Autodesk Inventor part; units mm, degrees
ref_plane "YZ Plane" through (0, 0, 0) normal (1, 0, 0) x (0, 1, 0)
ref_plane "XZ Plane" through (0, 0, 0) normal (0, 1, 0) x (-1, 0, 0)
ref_plane "XY Plane" through (0, 0, 0) normal (0, 0, 1) x (1, 0, 0)
sketch "Sketch1" plane through (0, 0, 0) normal (0, 1, 0) x (-1, 0, 0)
  line L0 (50, -20) -> (-50, -20)
  line L1 (-50, -20) -> (-50, 60)
  line L2 (-50, 60) -> (50, 60)
  line L3 (50, 60) -> (50, -20)
  point P0 (0, 0)
  dimension "d0" = 100
  dimension "d1" = 80
  dimension "d2" = 20
  dimension "d3" = 50
extrude "Plate1" add sketch "Sketch1" along normal blind 3
sketch "Sketch3" plane through (0, 3, 0) normal (0, 1, 0) x (1, 0, 0)
  circle A0 centre (9.405, -34) radius 1.05
  circle A1 centre (9.405, -6) radius 1.05
  circle A2 centre (0, -34) radius 1.05
  circle A3 centre (0, -6) radius 1.05
  circle A4 centre (-9.405, -34) radius 1.05
  circle A5 centre (-9.405, -6) radius 1.05
  line L0 (15.405, 0) -> (15.405, -40)
  line L1 (-15.405, -40) -> (15.405, -40)
  line L2 (-15.405, -40) -> (-15.405, 0)
  line L3 (15.405, 0) -> (-15.405, 0)
  point P0 (0, 0)
hole "Hole1" at (-9.405, 3, 6) at (0, 3, 6) at (9.405, 3, 6) at (9.405, 3, 34) at (0, 3, 34) at (-9.405, 3, 34) direction (0, -1, 0) diameter 2.1 depth 3 countersink diameter 4 countersink angle 90
equation "\"d20\" = Thickness"
equation "\"d4\" = Thickness"
equation "\"BendReliefWidth\" = Thickness"
equation "\"BendReliefDepth\" = 0.5 * Thickness"
equation "\"CornerReliefSize\" = 4 * Thickness"
equation "\"MinimumRemnant\" = 2 * Thickness"
equation "\"TransitionRadius\" = BendRadius"
equation "\"JacobiRadiusSize\" = BendRadius"
equation "\"GapSize\" = Thickness"
properties part number "axis_12_bottom_frame(bottom)" material "Aluminum 6061-AHC"
Input: part model. Units: mm. Frame: model coordinates. Coordinates: 2 decimals unless noted, no trailing zeros. Write each loop counter-clockwise with the first axis right and the second up, starting at its lowest first coordinate (ties: lowest second). Pieces come first, ordered by that corner, then holes. Notation, with made-up numbers: (14.25, 37.25) -> (67.25, 37.25) arc R22 cw to (67.25, 51.25) -> close; hole circle Ø10 at (-1.5, 51.25). An arc over 180 degrees is marked (long way). Write each question's results on one line, items separated by ' | '.
Item 1: Mould query, pull axis X, two halves, no side actions, for faces 1 (the flat face through (-50, 1, 21)), 2 (the cylindrical face through (10.43, 1.01, 5.77)), 3 (the flat face through (-1, 1, -20)), 4 (the cylindrical face through (-8.38, 1.01, 5.77)). Classes: +X half, -X half, draft (parallel to the pull), parting line (faces both ways), or undercut.
Conclusion:
face 1: -X half | face 2: undercut | face 3: draft | face 4: undercut
Item 2: Section query B-B on z = 34. Return loops of the section in (x, y) (3 decimals), plus the area to 3 significant figures.
Conclusion:
outline: (-50, 0) -> (-10.455, 0) -> (-10.455, 2.05) -> (-11.405, 3) -> (-50, 3) -> close; (-8.355, 0) -> (-1.05, 0) -> (-1.05, 2.05) -> (-2, 3) -> (-7.405, 3) -> (-8.355, 2.05) -> close; (1.05, 0) -> (8.355, 0) -> (8.355, 2.05) -> (7.405, 3) -> (2, 3) -> (1.05, 2.05) -> close; (10.455, 0) -> (50, 0) -> (50, 3) -> (11.405, 3) -> (10.455, 2.05) -> close | area: 278 mm^2
Item 3: Pin query (flat end, axial travel): pin 1 Ø2.5 at (x, z) = (9.405, 6) entering from +Y; pin 2 Ø1.3 at (x, z) = (0, 34) entering from +Y; pin 3 Ø3.5 at (x, z) = (0, 6) entering from +Y. Return the tip coordinate at first contact, or that it passes through.
Conclusion:
pin 1: stops at y = 2.25 | pin 2: passes through | pin 3: stops at y = 2.75
Item 4: Material intervals for probe 1 along Z at (x, y) = (0, 1.1); probe 2 along X at (y, z) = (0.4, 34) (3 decimals); probe 3 along Z at (x, y) = (-10.5, 2.4), sorted ascending.
Conclusion:
probe 1: z = -20 to 4.95, 7.05 to 32.95, 35.05 to 60 | probe 2: x = -50 to -10.455, -8.355 to -1.05, 1.05 to 8.355, 10.455 to 50 | probe 3: z = -20 to 5.13, 6.87 to 33.13, 34.87 to 60
Item 5: Section query A-A on x = 0. Return loops of the section in (y, z).
Conclusion:
outline: (0, -20) -> (3, -20) -> (3, 4) -> (2.05, 4.95) -> (0, 4.95) -> close; (0, 7.05) -> (2.05, 7.05) -> (3, 8) -> (3, 32) -> (2.05, 32.95) -> (0, 32.95) -> close; (0, 35.05) -> (2.05, 35.05) -> (3, 36) -> (3, 60) -> (0, 60) -> close
